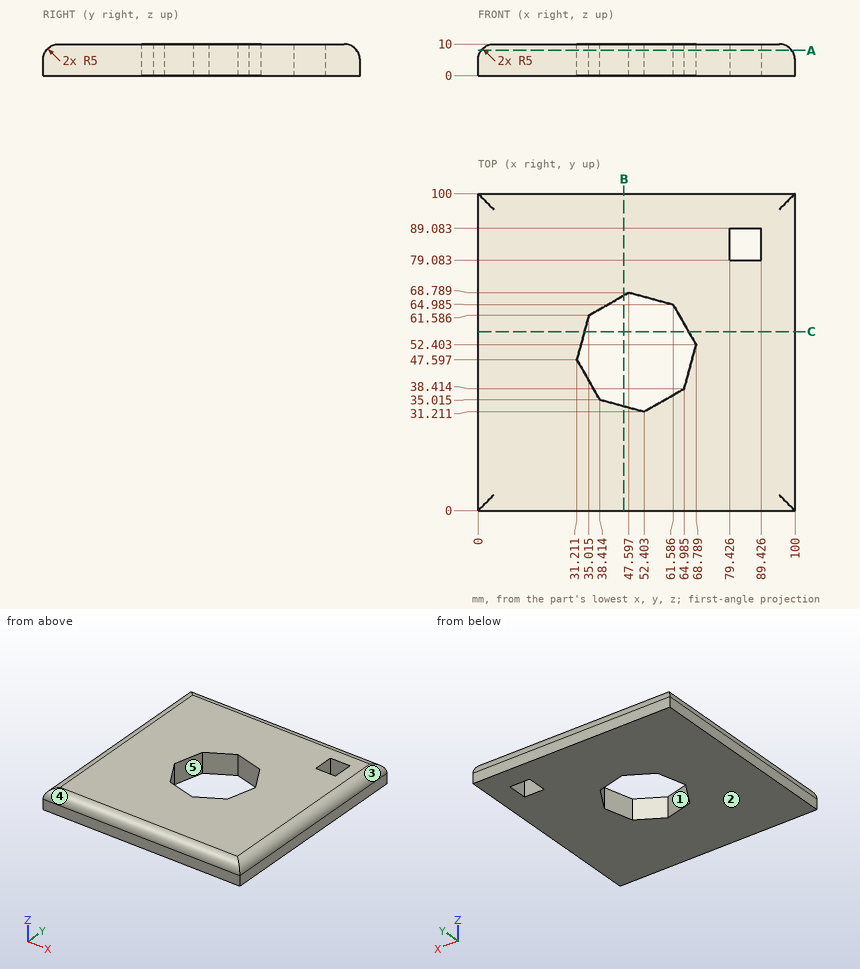
Drawing for the job (mm, zero at the part's lowest x, y, z). A direction names the side the tool comes from. Give positions to 0.01 mm unless a question says otherwise; leave off trailing zeros. Order: outer loops, then holes, each group sorted by start corner. A loop starts at its lowest first (then second) coordinate and runs counter-clockwise, first axis right, second up. Notation, with made-up numbers: (60, -28) - (68, -28) arc R32 ccw to (68, 0) - close; hole circle Ø4 at (43.25, -28.75). An arc over 180 degrees is marked (long way). Use one line per item in the form item = value.
Item 1: Pin check, flat tips, straight feed: pin 1 Ø3 at (x, z) = (84.5, 7) entering from +Y (1 decimal); pin 2 Ø5 at (y, z) = (60, 8) entering from -X (1 decimal). Stop position of each tip, or through.
Solution:
pin_1 = 100
pin_2 = 0
Item 2: Slice it at A-A on z = 8. Give the cut face in (x, y) (1 decimal).
Solution:
outline = (1, 1) - (99, 1) - (99, 99) - (1, 99) - close; hole (31.2, 47.6) - (38.4, 35) - (52.4, 31.2) - (65, 38.4) - (68.8, 52.4) - (61.6, 65) - (47.6, 68.8) - (35, 61.6) - close; hole (79.4, 79.1) - (89.4, 79.1) - (89.4, 89.1) - (79.4, 89.1) - close
Item 3: Two-plate mould, pull along X, no slides. Class the marked faces 3, 4 and 5: released by +X, released by -X, zero draft, split by the parting line, or undercut.
Solution:
face_3 = released by +X
face_4 = zero draft
face_5 = undercut
Item 4: Slice it at B-B on x = 46. Give the cut face in (y, z) (1 decimal).
Solution:
outline = (0, 0) - (33, 0) - (33, 10) - (5, 10) arc R5 ccw to (0, 5) - close; (67.9, 0) - (100, 0) - (100, 5) arc R5 ccw to (95, 10) - (67.9, 10) - close
Item 5: Slice it at C-C on y = 56.5. Give the cut face in (x, z).
Solution:
outline = (0, 0) - (33.63, 0) - (33.63, 10) - (5, 10) arc R5 ccw to (0, 5) - close; (66.44, 0) - (100, 0) - (100, 5) arc R5 ccw to (95, 10) - (66.44, 10) - close
Item 6: Probe probe 1 along Y at (x, z) = (79.5, 2.75); probe 2 along X at (y, z) = (88.5, 3.5); probe 3 along X at (y, z) = (40, 3.25) (1 decimal). List the from-to ranges inside material, lowest first. Write a range as from..to.
Solution:
probe_1 = 0..79.08, 89.08..100
probe_2 = 0..79.43, 89.43..100
probe_3 = 0..35.6, 65.4..100
Item 7: Which spindle directions (+Z, -Z, +X, -X, +Y, -Y) get a long thin tool onto all of the face, cutting with end or side? Do the marked faces 1 and 2. Say none if no direction does.
Solution:
face_1 = +Z, -Z
face_2 = -Z, +X, -X, +Y, -Y
